from build123d import *

# Parameters (mm, degrees)
EXTRUDE_1_DEPTH     = 6
SKETCH_2_R          = 1.5
SKETCH_2_R_2        = 3
CUT_EXTRUDE_1_DEPTH = 6
CUT_EXTRUDE_2_DEPTH = 2


with BuildPart() as part:
    # Эскиз1 → Бобышка-Вытянуть1 (new body)
    with BuildSketch(Plane(origin=(0, 0, 0), x_dir=(1, 0, 0), z_dir=(0, 1, 0))):
        with BuildLine():
            Line((17, -37), (-17, -37))
            ThreePointArc((-17, -37), (-31.142135624, -31.142135624), (-37, -17))
            Line((-37, -17), (-37, 17))
            ThreePointArc((-37, 17), (-31.142135624, 31.142135624), (-17, 37))
            Line((-17, 37), (17, 37))
            ThreePointArc((17, 37), (31.142135624, 31.142135624), (37, 17))
            Line((37, 17), (37, -17))
            ThreePointArc((37, -17), (31.142135624, -31.142135624), (17, -37))
        make_face()
    extrude(amount=EXTRUDE_1_DEPTH)

    # Эскиз2 → Вырез-Вытянуть1 (cut)
    with BuildSketch(Plane(origin=(0, 0, 0), x_dir=(1, 0, 0), z_dir=(0, 1, 0))):
        with Locations(Location((-27, 27, 0), (0, 0, 270))):
            Circle(SKETCH_2_R)
        with Locations(Location((27, 27, 0), (0, 0, 270))):
            Circle(SKETCH_2_R)
        with Locations(Location((27, -27, 0), (0, 0, 270))):
            Circle(SKETCH_2_R)
        with Locations(Location((-27, -27, 0), (0, 0, 270))):
            Circle(SKETCH_2_R)
        with Locations(Location((0, 0, 0), (0, 0, 270))):
            Circle(SKETCH_2_R_2)
    extrude(amount=CUT_EXTRUDE_1_DEPTH, mode=Mode.SUBTRACT)

    # Эскиз3 → Вырез-Вытянуть2 (cut)
    with BuildSketch(Plane(origin=(0, 0, 0), x_dir=(1, 0, 0), z_dir=(0, 1, 0))):
        Polygon((-28.732050808, 30), (-30.464101615, 27), (-28.732050808, 24), (-25.267949192, 24), (-23.535898385, 27), (-25.267949192, 30), align=None)
        Polygon((25.267949192, 30), (23.535898385, 27), (25.267949192, 24), (28.732050808, 24), (30.464101615, 27), (28.732050808, 30), align=None)
        Polygon((25.267949192, -24), (23.535898385, -27), (25.267949192, -30), (28.732050808, -30), (30.464101615, -27), (28.732050808, -24), align=None)
        Polygon((-28.732050808, -24), (-30.464101615, -27), (-28.732050808, -30), (-25.267949192, -30), (-23.535898385, -27), (-25.267949192, -24), align=None)
    extrude(amount=CUT_EXTRUDE_2_DEPTH, mode=Mode.SUBTRACT)


solid = part.part
Verification items for the finished model (mm, model axes). A direction names the side the tool comes from. Give positions to 0.01 mm unless a question says otherwise; leave off trailing zeros. Loops run counter-clockwise (first coordinate to the right, second up) from the corner with the lowest first, then second, coordinate; pieces in that order, holes last.
1) Set-up check for faces 1 (the flat face through (37, 3, 0)), 2 (the flat face through (27, 1, 24)): record each of +Z, -Z, +X, -X, +Y, -Y from which the full face is reachable in a straight line by a thin tool's end or side.
2) Draft check along X on faces 3 (the flat face through (24.4, 1, -25.5)), 4 (the cylindrical face through (30.986, 2.958, -31.297)), 5 (the cylindrical face through (-31.297, 2.958, -30.986)). Enter one of: pulls with the +X half, pulls with the -X half, needs draft (parallel to the pull), parting line crosses it, or undercut.
3) Sectioned sample at C-C, the plane x = 27. Enter the section's corners in (y, z).
4) Depth check by flat-ended pin: pin 1 Ø1 at (x, y) = (-27.5, 0.5) entering from +Z; pin 2 Ø3.5 at (x, z) = (27, -27) entering from -Y; pin 3 Ø0.6 at (x, y) = (-26.5, 1.5) entering from -Z. Enter the tip coordinate at first touch or a pass-through.
5) Sectioned sample at B-B, the plane y = 4.55. Enter the section's corners in (x, z), then the cut area to 3 significant figures.
6) Sectioned sample at A-A, the plane z = 0. Enter the section's corners in (x, y), then the cut area to 3 significant figures.
7) Thickness scan on line 1 along Z through (x, y) = (-27, 3.9); line 2 along X through (y, z) = (3.8, 0). Record the ranges inside material, lowest first.
Answers:
1. face 1: +Z, -Z, +X, +Y, -Y
1. face 2: -Y
2. face 3: undercut
2. face 4: pulls with the +X half
2. face 5: pulls with the -X half
3. outline: (0, -34.32) - (6, -34.32) - (6, -28.5) - (2, -28.5) - (2, -30) - (0, -30) - close; (0, -24) - (2, -24) - (2, -25.5) - (6, -25.5) - (6, 25.5) - (2, 25.5) - (2, 24) - (0, 24) - close; (0, 30) - (2, 30) - (2, 28.5) - (6, 28.5) - (6, 34.32) - (0, 34.32) - close
4. pin 1: stops at z = 34.32
4. pin 2: stops at y = 2
4. pin 3: stops at z = -34.76
5. outline: (-37, -17) arc R20 ccw to (-17, -37) - (17, -37) arc R20 ccw to (37, -17) - (37, 17) arc R20 ccw to (17, 37) - (-17, 37) arc R20 ccw to (-37, 17) - close; hole circle Ø3 at (-27, -27); hole circle Ø3 at (-27, 27); hole circle Ø6 at (0, 0); hole circle Ø3 at (27, -27); hole circle Ø3 at (27, 27)
5. area: 5,080 mm2
6. outline: (-37, 0) - (-3, 0) - (-3, 6) - (-37, 6) - close; (3, 0) - (37, 0) - (37, 6) - (3, 6) - close
6. area: 408 mm2
7. line 1: z = -34.32 to -28.5, -25.5 to 25.5, 28.5 to 34.32
7. line 2: x = -37 to -3, 3 to 37
